Verification items for the finished model (mm, model axes). Give positions to 0.01 mm unless a question says otherwise; leave off trailing zeros. Loops run counter-clockwise (first coordinate to the right, second up) from the corner with the lowest first, then second, coordinate; pieces in that order, holes last. Notation, with made-up numbers: (-1.75, 51) - (25.25, 51) arc R17 ccw to (25.25, 71) - close; hole circle Ø2 at (23, 57). An arc over 180 degrees is marked (long way). Use one line per item in the form item = value.
```python
from build123d import *

# Parameters (mm, degrees)
SKETCH_1_R          = 1.6
EXTRUDE_1_DEPTH     = 2
SKETCH_2_R          = 2.5
EXTRUDE_2_DEPTH     = 30
FILLET_1_R          = 0.5
SKETCH_3_R          = 0.75
CUT_EXTRUDE_1_DEPTH = 35.165040612
SKETCH_4_W          = 5.098076211
SKETCH_4_H          = 7
CUT_EXTRUDE_2_DEPTH = 34.841542518


with BuildPart() as part:
    # 草图1 → 凸台-拉伸1 (new body)
    with BuildSketch(Plane(origin=(0, 0, 0), x_dir=(1, 0, 0), z_dir=(0, 1, 0))):
        with BuildLine():
            Line((3, 0), (12.5, 0))
            Line((12.5, 0), (12.5, -30))
            Line((12.5, -30), (3, -30))
            ThreePointArc((3, -30), (0.878679656, -29.121320344), (0, -27))
            Line((0, -27), (0, -3))
            ThreePointArc((0, -3), (0.878679656, -0.878679656), (3, 0))
        make_face()
        with Locations(Location((4.5, -5, 0), (0, 0, 270))):
            Circle(SKETCH_1_R, mode=Mode.SUBTRACT)
        with Locations(Location((4.5, -25, 0), (0, 0, 270))):
            Circle(SKETCH_1_R, mode=Mode.SUBTRACT)
    extrude(amount=EXTRUDE_1_DEPTH)

    # 草图2 → 凸台-拉伸2 (add)
    with BuildSketch(Plane.XY.offset(30)):
        with Locations((12.5, 4)):
            Circle(SKETCH_2_R)
    extrude(amount=-EXTRUDE_2_DEPTH)

    # 圆角1
    fillet_1_edges = [part.edges().sort_by_distance(p)[0] for p in [
        (12.5, 1.5, 15),
        (11, 2, 15),
        (12.5, 0, 15),
    ]]
    fillet(fillet_1_edges, radius=FILLET_1_R)

    # 草图3 → 切除-拉伸1 (cut, through all)
    with BuildSketch(Plane.XY.offset(30)):
        with Locations((12.5, 4)):
            Circle(SKETCH_3_R)
    extrude(amount=-CUT_EXTRUDE_1_DEPTH, mode=Mode.SUBTRACT)

    # 草图4 → 切除-拉伸2 (cut, through all)
    with BuildSketch(Plane(origin=(0, 2, 0), x_dir=(1, 0, 0), z_dir=(0, 1, 0))):
        with Locations((12.450961895, -3.5)):
            Rectangle(SKETCH_4_W, SKETCH_4_H)
        with Locations((12.450961895, -26.5)):
            Rectangle(SKETCH_4_W, SKETCH_4_H)
    extrude(amount=CUT_EXTRUDE_2_DEPTH, mode=Mode.SUBTRACT)


solid = part.part
```
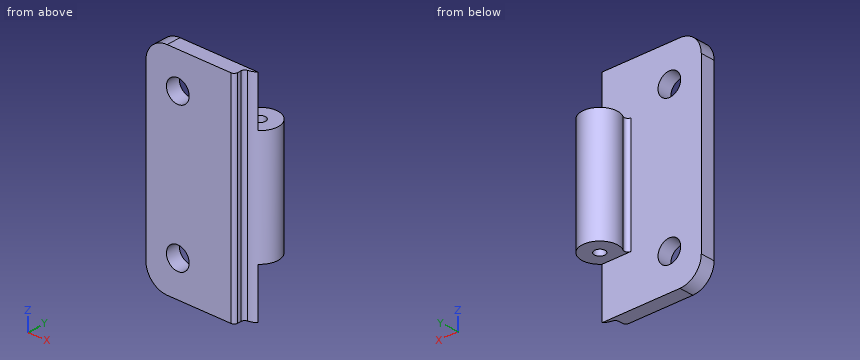
1. Section check C-C, the plane x = 4.5. Record the cut outline in (y, z).
Result set:
outline = (0, 0) - (2, 0) - (2, 3.4) - (0, 3.4) - close; (0, 6.6) - (2, 6.6) - (2, 23.4) - (0, 23.4) - close; (0, 26.6) - (2, 26.6) - (2, 30) - (0, 30) - close
2. Depth check by flat-ended pin: pin 1 Ø5 at (x, z) = (4.5, 5) entering from -Y; pin 2 Ø1 at (y, z) = (3, 19.5) entering from +X; pin 3 Ø4 at (x, z) = (1.5, 13.5) entering from +Y; pin 4 Ø1.5 at (x, y) = (10.5, 5) entering from +Z. Enter the tip coordinate at first touch or a pass-through.
Result set:
pin_1 = 0
pin_2 = 14.95
pin_3 = 2
pin_4 = 23
3. Section check B-B, the plane z = 25. Record the cut outline in (x, y), then the cut area to 3 significant figures.
Result set:
outline = (0, 0) - (2.9, 0) - (2.9, 2) - (0, 2) - close; (6.1, 0) - (12, 0) arc R0.5 ccw to (12.5, 0.5) - (12.5, 1.04) arc R0.5 cw to (12.92, 1.53) arc R2.5 ccw to (14, 2) - (6.1, 2) - close
area = 19.1 mm²
4. Scan lines: probe 1 along X at (y, z) = (0.75, 5); probe 2 along Y at (x, z) = (11.75, 4); probe 3 along Z at (x, y) = (13.5, 3.25). Record each from-to range of solid material in increasing order.
Result set:
probe_1 = 0 to 2.9, 6.1 to 12.5
probe_2 = 0 to 2
probe_3 = 7 to 23
5. Section check A-A, the plane y = 4. Record the cut outline in (x, z), then the cut area to 3 significant figures.
Result set:
outline = (10, 7) - (11.75, 7) - (11.75, 23) - (10, 23) - close; (13.25, 7) - (15, 7) - (15, 23) - (13.25, 23) - close
area = 56.0 mm²
6. Section check D-D, the plane x = 7.5. Record the cut outline in (y, z).
Result set:
outline = (0, 0) - (2, 0) - (2, 30) - (0, 30) - close
